Could you check a few things on this model? Use its own coordinates, in mm. A direction names the side the tool comes from. Give positions to 0.01 mm unless a question says otherwise; leave off trailing zeros. Return JSON: item names as keys, results as strings. Group by question number.
1. Please list where these lines run through material, in increasing order: line 1 (Z direction, x = 4.75, y = -2.5); line 2 (Y direction, x = 3.75, z = 8); line 3 (Y direction, x = 0.9, z = 0).
2. For faces 4 (the cylindrical face through (2.22, -15.11, -1.98)), 5 (the cylindrical face through (3.014, 18.597, -4.13)), 6 (the cylindrical face through (4.95, -15.11, -1.98)), which set-ups out of +Z, -Z, +X, -X, +Y, -Y let a thin tool reach every point of the face, with its end or its side?
3. If we mould it in two halves opening along X, with no side actions, what happens to faces 1 (the flat face through (5.461, 4.4, -13.5)), 2 (the cylindrical face through (1.03, 13.576, -3.015)), 3 (the flat face through (2.032, 10, 12))? For each: +X half, -X half, draft (parallel to the pull), parting line (faces both ways), or undercut.
4. For pin 1 (20.5 mm diameter, centred on y = 0, z = 0, fed in from -X); pin 2 (17 mm diameter, centred on y = 5.5, z = -8, fed in from +X); pin 3 (3 mm diameter, centred on x = 2, y = 13, fed in from +Z); pin 4 (1.5 mm diameter, centred on x = 4, z = 13.5, fed in from -Y), each with a flat end and sliding along its axis, tell me the tip position at first contact or that it passes through.
```python
from build123d import *

# Parameters (mm, degrees)
EDGE_FILLET_R = 0.635


with BuildPart() as part:
    # Primary Sketch → Primary Revolve (revolve)
    with BuildSketch(Plane.XY, mode=Mode.PRIVATE) as primary_revolve_sk:
        with BuildLine():
            Line((2.032, 17.145), (6.096, 17.145))
            Line((6.096, 17.145), (6.096, 19.05))
            Line((6.096, 19.05), (0, 19.05))
            Line((0, 19.05), (0, 17.145))
            Line((0, 17.145), (0, 13.9065))
            Line((0, 13.9065), (2.032, 13.9065))
            Line((2.032, 13.9065), (3.429, 12.5095))
            Line((3.429, 12.5095), (4.826, 13.9065))
            Line((4.826, 13.9065), (5.461, 13.9065))
            Line((5.461, 13.9065), (5.461, 15.24))
            Line((5.461, 15.24), (4.445, 15.24))
            ThreePointArc((4.445, 15.24), (3.429, 16.256), (2.413, 15.24))
            Line((2.413, 15.24), (2.032, 15.24))
            Line((2.032, 15.24), (2.032, 17.145))
        make_face()
    revolve(primary_revolve_sk.sketch.rotate(Axis((0, 0, 0), (1, 0, 0)), 90), axis=Axis((0, 0, 0), (1, 0, 0)))

    # Edge Fillet
    edge_fillet_edges = [part.edges().sort_by_distance(p)[0] for p in [
        (6.096, 0, -19.05),
        (0, 0, -19.05),
    ]]
    fillet(edge_fillet_edges, radius=EDGE_FILLET_R)


solid = part.part
```
Answer:
{
 "1": {"line 1": "z = -18.89 to -16.96, -15.03 to -13.6, 13.6 to 15.03, 16.96 to 18.89", "line 2": "y = -17.29 to -15.16, -14.09 to -10.03, 10.03 to 14.09, 15.16 to 17.29", "line 3": "y = -19.05 to -13.91, 13.91 to 19.05"},
 "2": {"face 4": "none", "face 5": "+X, -X", "face 6": "+X"},
 "3": {"face 1": "+X half", "face 2": "draft", "face 3": "undercut"},
 "4": {"pin 1": "passes through", "pin 2": "stops at x = 6.1", "pin 3": "stops at z = 15.19", "pin 4": "stops at y = -14.15"}
}
